```python
from build123d import *

# Parameters (mm, degrees)
CROQUIS1_W              = 35
CROQUIS1_H              = 35
CROQUIS1_W_2            = 31
CROQUIS1_H_2            = 31
SALIENTE_EXTRUIR1_DEPTH = 1000
CROQUIS2_R              = 4
CORTAR_EXTRUIR1_DEPTH   = 35
CROQUIS3_R              = 4
CORTAR_EXTRUIR2_DEPTH   = 35


with BuildPart() as part:
    # Croquis1 → Saliente-Extruir1 (new body)
    with BuildSketch(Plane(origin=(0, 0, 0), x_dir=(1, 0, 0), z_dir=(0, 1, 0))):
        with Locations((17.5, 17.5)):
            Rectangle(CROQUIS1_W, CROQUIS1_H)
        with Locations((17.5, 17.5)):
            Rectangle(CROQUIS1_W_2, CROQUIS1_H_2, mode=Mode.SUBTRACT)
    extrude(amount=SALIENTE_EXTRUIR1_DEPTH)

    # Croquis2 → Cortar-Extruir1 (cut)
    with BuildSketch(Plane.XY):
        with Locations((17.5, 20)):
            Circle(CROQUIS2_R)
    extrude(amount=-CORTAR_EXTRUIR1_DEPTH, mode=Mode.SUBTRACT)

    # Croquis3 → Cortar-Extruir2 (cut)
    with BuildSketch(Plane(origin=(0, 0, -35), x_dir=(-1, 0, 0), z_dir=(0, 0, -1))):
        with Locations((-17.5, 979)):
            Circle(CROQUIS3_R)
    extrude(amount=-CORTAR_EXTRUIR2_DEPTH, mode=Mode.SUBTRACT)


solid = part.part
```
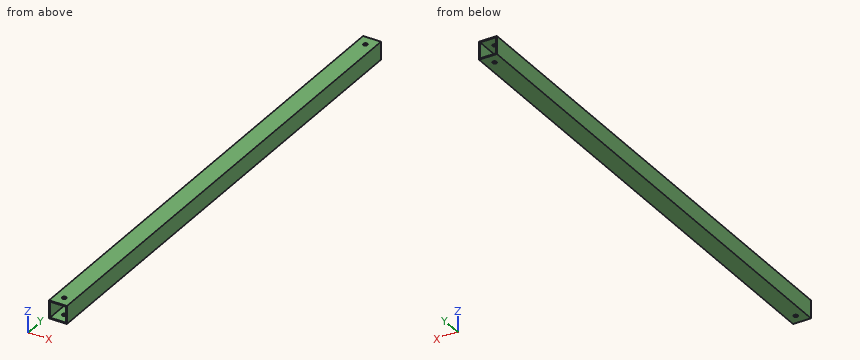
Could you check a few things on this model? Use its own coordinates, in mm. Round coordinates to 2 decimals unless told otherwise and drop trailing zeros. Loops run counter-clockwise (first coordinate to the right, second up) from the corner with the lowest first, then second, coordinate; pieces in that order, holes last. Notation, with made-up numbers: (80, 79) - (96, 79) arc R24 cw to (96, 106) - close; hole circle Ø9 at (26, 79). An arc over 180 degrees is marked (long way). Answer as CSV lines item,"result".
1. For pin 1 Ø5 at (x, y) = (17.5, 979) entering from -Z, with a flat end and sliding along its axis, tell me the tip position at first contact or that it passes through.
Filled in:
pin 1,"passes through"
2. Please list where these lines run through material, in increasing order: line 1 along Y through (x, z) = (17.5, -34.45); line 2 along X through (y, z) = (802.5, -9); line 3 along X through (y, z) = (979, -0.5). Write a range as [from, to].
Filled in:
line 1,"y = [0, 16], [24, 975], [983, 1000]"
line 2,"x = [0, 2], [33, 35]"
line 3,"x = [0, 13.5], [21.5, 35]"
3. I want a section at A-A on y = 227.5. List the corners of the cut face in (x, z) for me.
Filled in:
outline,"(0, -35) - (35, -35) - (35, 0) - (0, 0) - close; hole (2, -33) - (33, -33) - (33, -2) - (2, -2) - close"
4. I want a section at B-B on z = -10.5. List the corners of the cut face in (x, y) for me, then the cut area to 3 significant figures.
Filled in:
outline,"(0, 0) - (2, 0) - (2, 1000) - (0, 1000) - close; (33, 0) - (35, 0) - (35, 1000) - (33, 1000) - close"
area,"4,000 mm^2"
